from build123d import *

# Parameters (mm, degrees)
F1_DEPTH = 63.5
F2_DEPTH = 25.4
F3_DEPTH = 20.6375
F5_R     = 5.08


with BuildPart() as f1:
    # F0 (on Front) → F1 (new body, symmetric)
    with BuildSketch(Plane.XZ):
        Polygon((-41.275, -9.525), (41.275, -9.525), (41.275, 9.525), (22.225, 9.525), (-41.275, 9.525), align=None)
    extrude(amount=F1_DEPTH, both=True)

    # F0 (on Front) → F2 (join, symmetric)
    with BuildSketch(Plane.XZ):
        with BuildLine():
            Line((22.225, 9.525), (41.275, 9.525))
            Line((41.275, 9.525), (41.275, 27.0002))
            ThreePointArc((41.275, 27.0002), (45.9246798487, 38.2255201513), (57.15, 42.8752))
            Line((57.15, 42.8752), (75.8391746044, 42.8752))
            Line((75.8391746044, 42.8752), (75.8391746044, 61.9252))
            Line((75.8391746044, 61.9252), (72.1653963261, 61.9252))
            Line((72.1653963261, 61.9252), (64.4478433083, 61.9252))
            add(Edge.make_bspline(
                [(51.5934381261, 61.4803427657), (55.8377621911, 61.7230212557), (60.1301345398, 61.8704467699), (64.4478433083, 61.9252)],
                knots=[109.9989727247, 109.9989727247, 109.9989727247, 109.9989727247, 119.3829591055, 119.3829591055, 119.3829591055, 119.3829591055], degree=3))
            ThreePointArc((51.5934381261, 61.4803427657), (30.5622345011, 49.6463111623), (22.225, 27.0002))
            Line((22.225, 27.0002), (22.225, 9.525))
        make_face()
    extrude(amount=F2_DEPTH, both=True)

    # F0 (on Front) → F3 (join, symmetric)
    with BuildSketch(Plane.XZ):
        with BuildLine():
            add(Edge.make_bspline(
                [(-41.275, 9.525), (-41.3083164925, 42.7027595487), (1.841523734, 58.6356684957), (51.5934381261, 61.4803427657)],
                knots=[0, 0, 0, 0, 109.9989727247, 109.9989727247, 109.9989727247, 109.9989727247], degree=3))
            Line((-41.275, 9.525), (22.225, 9.525))
            Line((22.225, 9.525), (22.225, 27.0002))
            ThreePointArc((22.225, 27.0002), (30.5622345011, 49.6463111623), (51.5934381261, 61.4803427657))
        make_face()
    extrude(amount=F3_DEPTH, both=True)

    # F0 (on Front) → F4 (revolve)
    with BuildSketch(Plane.XZ):
        Polygon((87.1807926523, 66.675), (87.3169004917, 38.1), (126.6391746044, 38.1), (126.6391746044, 66.675), align=None)
    revolve(axis=Axis((87.248846572, 0, 52.3875), (-0.004763125, 0, 0.9999886563)))

    # F5
    f5_edges = [f1.edges().sort_by_distance(p)[0] for p in [
        (41.275, -63.5, 0),
        (-41.275, -63.5, 0),
        (41.275, 63.5, 0),
        (-41.275, 63.5, 0),
    ]]
    fillet(f5_edges, radius=F5_R)


solid = f1.part
Could you check a few things on this model? Use its own coordinates, in mm. A direction names the side the tool comes from. Give positions to 0.01 mm unless a question says otherwise; leave off trailing zeros. Order: outer loops, then holes, each group sorted by start corner. A loop starts at its lowest first (then second) coordinate and runs counter-clockwise, first axis right, second up. Notation, with made-up numbers: (42, 14) -> (53, 14) arc R19 cw to (53, 48) -> close; hole circle Ø9 at (82.25, 40.25). An arc over 180 degrees is marked (long way). Answer in a Markdown table with one row per item. Add a question column.
Item 1: I'm going to push flat-ended pins straight in: P1, Ø2, axis at x = 51, y = -21, coming from the -Z side; P2, Ø1, axis at x = 13, z = 22, coming from the +Y side; P3, Ø18.5, axis at y = -1, z = 9, coming from the +X side (3 decimals). Where does each tip first touch, or does it pass through?
Item 2: Imagine slicing it at B-B (y = -48). List the corners of the cut face in (x, z) for me (3 decimals).
Item 3: Imagine slicing it at A-A (z = 5). List the corners of the cut face in (x, y) for me (3 decimals).
Item 4: Please list where these lines run through material, in increasing order: probe 1 along Z at (x, y) = (17.5, 11) (3 decimals); probe 2 along X at (y, z) = (-5.5, 1) (3 decimals); probe 3 along Z at (x, y) = (29.5, -31) (3 decimals).
Item 5: We'd pull the mould along X, two halves only. Please class faces 1 (the flat face through (22.225, -23, 18)), 2 (the cylindrical face through (44.047, -0.356, 35.962)), 3 (the flat face through (-1, -63.5, 0)): pulls with the +X half, pulls with the -X half, needs draft (parallel to the pull), parting line crosses it, or undercut.
Item 6: For faces 4 (the flat face through (22.225, 23, 18)), 5 (the flat face through (41.275, -1, 4)), 6 (the cylindrical face through (30.79, -23.05, 49.91)), which set-ups out of +Z, -Z, +X, -X, +Y, -Y let a thin tool reach every point of the face, with its end or its side?
Result:
| question | item | result |
|---|---|---|
| 1 | P1 | z = 41.17 |
| 1 | P2 | y = 20.64 |
| 1 | P3 | x = 41.275 |
| 2 | outline | (-41.275, -9.525) -> (41.275, -9.525) -> (41.275, 9.525) -> (-41.275, 9.525) -> close |
| 3 | outline | (-41.275, -58.42) arc R5.08 ccw to (-36.195, -63.5) -> (36.195, -63.5) arc R5.08 ccw to (41.275, -58.42) -> (41.275, 58.42) arc R5.08 ccw to (36.195, 63.5) -> (-36.195, 63.5) arc R5.08 ccw to (-41.275, 58.42) -> close |
| 4 | probe 1 | -9.525 to 57.13 |
| 4 | probe 2 | -41.275 to 41.275 |
| 4 | probe 3 | -9.525 to 9.525 |
| 5 | face 1 | pulls with the -X half |
| 5 | face 2 | undercut |
| 5 | face 3 | needs draft |
| 6 | face 4 | +Z, -X, +Y |
| 6 | face 5 | -Z, +X, +Y, -Y |
| 6 | face 6 | +Z, -X, -Y |
